```python
from build123d import *

# Parameters (mm, degrees)
SKETCH1_W           = 104.902
SKETCH1_H           = 16.764
BOSS_EXTRUDE1_DEPTH = 5.334
SKETCH2_W           = 26.2255
SKETCH2_H           = 5.334
CUT_EXTRUDE1_DEPTH  = 59.030232747
FILLET1_R           = 6.35


with BuildPart() as part:
    # Sketch1 → Boss-Extrude1 (new body)
    with BuildSketch(Plane.XY):
        with Locations((-4.604300362, -0.769451102)):
            Rectangle(SKETCH1_W, SKETCH1_H)
    extrude(amount=BOSS_EXTRUDE1_DEPTH)

    # Sketch2 → Cut-Extrude1 (cut, through all)
    with BuildSketch(Plane.XY.offset(5.334)):
        with Locations((-43.942550362, -6.484451102)):
            Rectangle(SKETCH2_W, SKETCH2_H)
        with Locations((8.508449638, -6.484451102)):
            Rectangle(SKETCH2_W, SKETCH2_H)
    extrude(amount=-CUT_EXTRUDE1_DEPTH, mode=Mode.SUBTRACT)

    # Fillet1
    fillet1_edges = [part.edges().sort_by_distance(p)[0] for p in [
        (-57.055300362, 7.612548898, 2.667),
        (47.846699638, 7.612548898, 2.667),
    ]]
    fillet(fillet1_edges, radius=FILLET1_R)


solid = part.part
```
Design review of the part built by this model. Coordinates are the model's own, in mm. A direction names the side the tool comes from. Give positions to 0.01 mm unless a question says otherwise; leave off trailing zeros. Loops run counter-clockwise (first coordinate to the right, second up) from the corner with the lowest first, then second, coordinate; pieces in that order, holes last. Notation, with made-up numbers: (-10, 77) -> (45, 77) arc R17 cw to (45, 110) -> close; hole circle Ø10 at (27, -23.5). An arc over 180 degrees is marked (long way). One line per item, written item: value.
Q1. For pin 1 Ø1.6 at (x, z) = (15, 3.5) entering from -Y; pin 2 Ø2 at (x, y) = (-41.5, -1) entering from -Z; pin 3 Ø1.6 at (y, z) = (-6, 3.5) entering from -X, all flat-tipped, find the tip position at first contact; note any pin that passes through.
Numbers:
pin 1: stops at y = -3.82
pin 2: stops at z = 0
pin 3: stops at x = -30.83
Q2. We need section A-A on y = -6.5. Give the boundary of the cut face in (x, z), and give its area (3 significant figures).
Numbers:
outline: (-30.83, 0) -> (-4.6, 0) -> (-4.6, 5.33) -> (-30.83, 5.33) -> close; (21.62, 0) -> (47.85, 0) -> (47.85, 5.33) -> (21.62, 5.33) -> close
area: 280 mm^2
Q3. Draft analysis for pull direction Z (two halves, no side actions). For faces 1 (the flat face through (-5, 1, 5.334)), 2 (the cylindrical face through (-55.245, 5.703, 2.704)), 3 (the flat face through (-5, 1, 0)), state which applies: pulls with the +Z half, pulls with the -Z half, needs draft (parallel to the pull), parting line crosses it, or undercut.
Numbers:
face 1: pulls with the +Z half
face 2: needs draft
face 3: pulls with the -Z half
Q4. We need section C-C on x = -44. Give the boundary of the cut face in (y, z), and give its area (3 significant figures).
Numbers:
outline: (-3.82, 0) -> (7.61, 0) -> (7.61, 5.33) -> (-3.82, 5.33) -> close
area: 61.0 mm^2
Q5. We need section B-B on z = 1.6. Give the boundary of the cut face in (x, y), and give its area (3 significant figures).
Numbers:
outline: (-57.06, -3.82) -> (-30.83, -3.82) -> (-30.83, -9.15) -> (-4.6, -9.15) -> (-4.6, -3.82) -> (21.62, -3.82) -> (21.62, -9.15) -> (47.85, -9.15) -> (47.85, 1.26) arc R6.35 ccw to (41.5, 7.61) -> (-50.71, 7.61) arc R6.35 ccw to (-57.06, 1.26) -> close
area: 1,460 mm^2
Q6. We need section D-D on y = 4.5. Give the boundary of the cut face in (x, z), and give its area (3 significant figures).
Numbers:
outline: (-56.17, 0) -> (46.96, 0) -> (46.96, 5.33) -> (-56.17, 5.33) -> close
area: 550 mm^2
Q7. Machinability: for faces 4 (the flat face through (-30.83, -7, 3)), 5 (the flat face through (-4.604, -7, 3)), 6 (the flat face through (-18, -9.151, 3)), which of the approach directions +Z, -Z, +X, -X, +Y, -Y give a long, thin tool a straight path to every point of the face, cutting with its end or side? Answer none if there is none.
Numbers:
face 4: +Z, -Z, -X, -Y
face 5: +Z, -Z, -Y
face 6: +Z, -Z, +X, -X, -Y
Q8. For L1, parallel to X at y = -4.25, z = 3.6; L2, parallel to Y at x = 1, z = 2.55; L3, parallel to X at y = 7, z = 4.9, list the stretches that pass through material, from the lowest coordinate up.
Numbers:
L1: x = -30.83 to -4.6, 21.62 to 47.85
L2: y = -3.82 to 7.61
L3: x = -53.43 to 44.22
